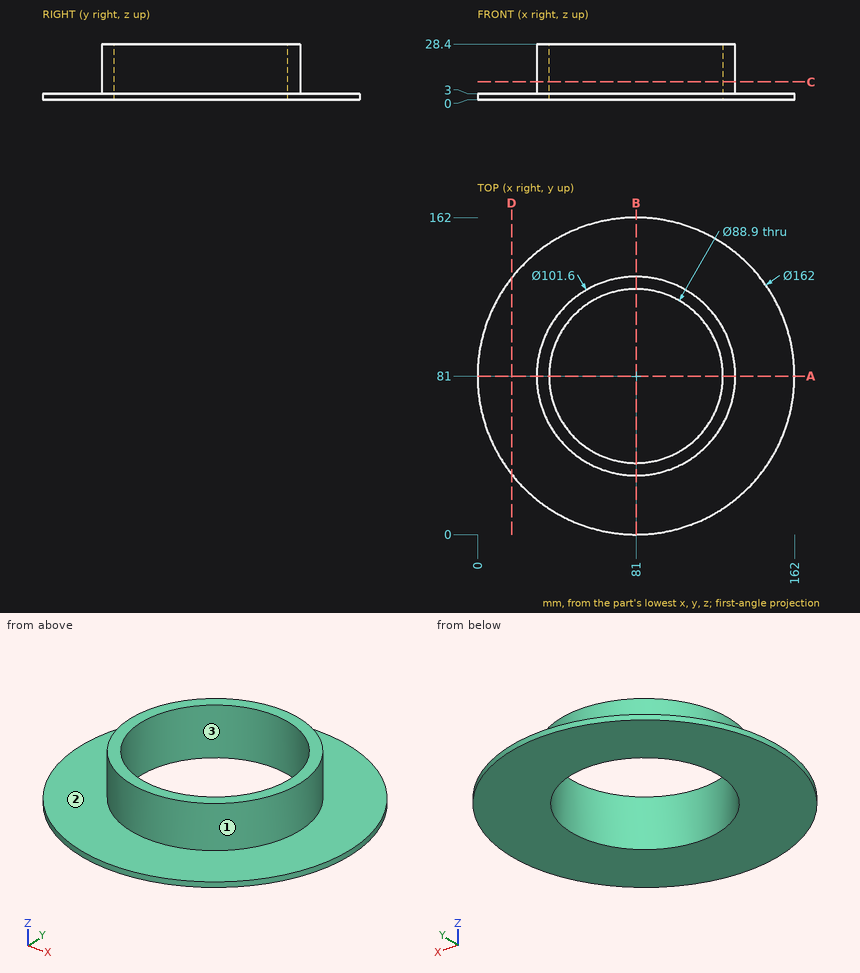
Source: three-view drawing plus pictorial views. Frame: mm from the lowest corner of the part. Round coordinates to 2 decimals unless told otherwise and drop trailing zeros. Write each loop counter-clockwise with the first axis right and the second up, starting at its lowest first coordinate (ties: lowest second). Pieces come first, ordered by that corner, then holes. Notation, with made-up numbers: M 1,7 L 35,7 A19 cw 35,44 Z; hole C 17.25,-36 d7. An arc over 180 degrees is marked long. One line per item, written item: value. Start each with the question number.
Item 1: Section query A-A (y = 81). Return the cut outline in (x, z), plus the area to 3 significant figures.
Item 2: Ray query, L1, parallel to Y at x = 81, z = 13; L2, parallel to Z at x = 31, y = 105; L3, parallel to Y at x = 95, z = 17.75. Return the intervals inside material, ascending. Write a range as from..to.
Item 3: Pin query (flat end, axial travel): pin 1 (1 mm diameter, centred on x = 79, z = 12.5, fed in from -Y); pin 2 (12 mm diameter, centred on x = 121.5, z = 6, fed in from +Y); pin 3 (1.5 mm diameter, centred on y = 39, z = 22, fed in from +X); pin 4 (1 mm diameter, centred on x = 26.5, y = 113.5, fed in from -Z). Return the tip coordinate at first contact, or that it passes through.
Item 4: Mould query, pull axis X, two halves, no side actions, for the marked faces 1, 2 and 3. Classes: pulls with the +X half, pulls with the -X half, needs draft (parallel to the pull), parting line crosses it, or undercut.
Item 5: Section query C-C (z = 9). Return the cut outline in (x, y), plus the area to 3 significant figures.
Item 6: Section query D-D (x = 17.5). Return the cut outline in (y, z), plus the area to 3 significant figures.
Result set:
1. outline: M 0,0 L 36.55,0 L 36.55,28.4 L 30.2,28.4 L 30.2,3 L 0,3 Z; M 125.45,0 L 162,0 L 162,3 L 131.8,3 L 131.8,28.4 L 125.45,28.4 Z
1. area: 542 mm²
2. L1: y = 30.2..36.55, 125.45..131.8
2. L2: z = 0..3
2. L3: y = 32.17..38.81, 123.19..129.83
3. pin 1: stops at y = 30.22
3. pin 2: stops at y = 153.9
3. pin 3: stops at x = 110.65
3. pin 4: stops at z = 0
4. face 1: parting line crosses it
4. face 2: needs draft
4. face 3: undercut
5. outline: C 81,81 d101.6; hole C 81,81 d88.9
5. area: 1,900 mm²
6. outline: M 30.71,0 L 131.29,0 L 131.29,3 L 30.71,3 Z
6. area: 302 mm²
